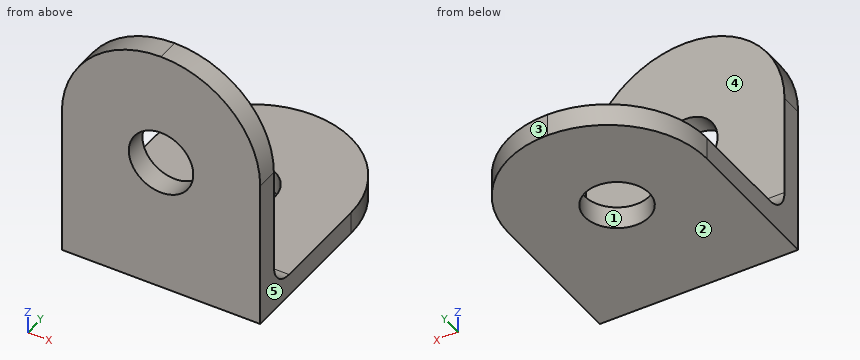
```python
from build123d import *

# Parameters (mm, degrees)
SKETCH1_W           = 16
SKETCH1_H           = 20
BOSS_EXTRUDE1_DEPTH = 1.8
SKETCH2_W           = 16
SKETCH2_H           = 18.2
BOSS_EXTRUDE2_DEPTH = 1.8
SKETCH3_R           = 2.6
CUT_EXTRUDE1_DEPTH  = 1.8
SKETCH4_R           = 2.6
CUT_EXTRUDE2_DEPTH  = 1.8
FILLET1_R           = 2
FILLET2_R           = 8


with BuildPart() as part:
    # Sketch1 → Boss-Extrude1 (new body)
    with BuildSketch(Plane.XY):
        with Locations((8, 10)):
            Rectangle(SKETCH1_W, SKETCH1_H)
    extrude(amount=BOSS_EXTRUDE1_DEPTH)

    # Sketch2 → Boss-Extrude2 (add)
    with BuildSketch(Plane.XZ):
        with Locations((8, 10.9)):
            Rectangle(SKETCH2_W, SKETCH2_H)
    extrude(amount=-BOSS_EXTRUDE2_DEPTH)

    # Sketch3 → Cut-Extrude1 (cut)
    with BuildSketch(Plane.XY.offset(1.8)):
        with Locations((8, 10.8)):
            Circle(SKETCH3_R)
    extrude(amount=-CUT_EXTRUDE1_DEPTH, mode=Mode.SUBTRACT)

    # Sketch4 → Cut-Extrude2 (cut)
    with BuildSketch(Plane(origin=(0, 1.8, 0), x_dir=(1, 0, 0), z_dir=(0, 1, 0))):
        with Locations(Location((8, -10.8, 0), (0, 0, 270))):
            Circle(SKETCH4_R)
    extrude(amount=-CUT_EXTRUDE2_DEPTH, mode=Mode.SUBTRACT)

    # Fillet1
    fillet1_edges = [part.edges().sort_by_distance(p)[0] for p in [
        (8, 1.8, 1.8),
    ]]
    fillet(fillet1_edges, radius=FILLET1_R)

    # Fillet2
    fillet2_edges = [part.edges().sort_by_distance(p)[0] for p in [
        (16, 0.9, 20),
        (0, 0.9, 20),
        (16, 20, 0.9),
        (0, 20, 0.9),
    ]]
    fillet(fillet2_edges, radius=FILLET2_R - 0.0001)  # a hair under: the kernel refuses the full size


solid = part.part
```
Build history of the part. All positions in model axes, mm. Face numbers are marked on the shaded views. A direction names the side the tool comes from. Round coordinates to 2 decimals unless told otherwise and drop trailing zeros. Write each loop counter-clockwise with the first axis right and the second up, starting at its lowest first coordinate (ties: lowest second). Pieces come first, ordered by that corner, then holes.
1) Drill centre lines: probe 1 along Y at (x, z) = (8, 1); probe 2 along Z at (x, y) = (11.75, 18). Where is each one in solid material? Low to high.
2) Band-saw the part on C-C, the plane x = 3.5. List the corners of the cut face in (y, z), and give its area (3 significant figures).
3) Band-saw the part on D-D, the plane z = 4.5. List the corners of the cut face in (x, y).
4) Mould opens along X. For the marked faces 1, 2 and 3 say: +X half, -X half, draft (parallel to the pull), parting line (faces both ways), or undercut.
5) 3-axis set-ups, long thin cutter, end or side, ignore diameter. For the marked faces 4 and 5: which of +Z, -Z, +X, -X, +Y, -Y reach the whole face in a straight line?
6) Band-saw the part on A-A, the plane z = 10.8. List the corners of the cut face in (x, y).
7) Pin check, flat tips, straight feed: pin 1 (3 mm diameter, centred on x = 13.5, y = 14, fed in from +Z); pin 2 (3 mm diameter, centred on x = 3.5, z = 6, fed in from +Y); pin 3 (3 mm diameter, centred on x = 8, y = 10.8, fed in from -Z). Stop position of each tip, or through.
Ans:
1. probe 1: y = 0 to 8.2, 13.4 to 20
1. probe 2: z = 0 to 1.8
2. outline: (0, 0) - (18.61, 0) - (18.61, 1.8) - (3.8, 1.8) arc R2 cw to (1.8, 3.8) - (1.8, 18.61) - (0, 18.61) - close
2. area: 64.6 mm2
3. outline: (0, 0) - (16, 0) - (16, 1.8) - (0, 1.8) - close
4. face 1: undercut
4. face 2: draft
4. face 3: +X half
5. face 4: +Z, +X, -X, +Y
5. face 5: +Z, -Z, +X, +Y, -Y
6. outline: (0, 0) - (5.4, 0) - (5.4, 1.8) - (0, 1.8) - close; (10.6, 0) - (16, 0) - (16, 1.8) - (10.6, 1.8) - close
7. pin 1: stops at z = 1.8
7. pin 2: stops at y = 1.8
7. pin 3: passes through
